Autodesk Inventor part; units mm, degrees
ref_plane "YZ Plane" through (0, 0, 0) normal (1, 0, 0) x (0, 1, 0)
ref_plane "XZ Plane" through (0, 0, 0) normal (0, 1, 0) x (-1, 0, 0)
ref_plane "XY Plane" through (0, 0, 0) normal (0, 0, 1) x (1, 0, 0)
sketch "Sketch1" plane through (0, 0, 0) normal (0, 1, 0) x (-1, 0, 0)
  line L0 (9.98, 16.98) -> (-9.98, 16.98)
  line L1 (-9.98, 16.98) -> (-9.98, -16.98)
  line L2 (-9.98, -16.98) -> (9.98, -16.98)
  line L3 (9.98, -16.98) -> (9.98, 16.98)
  line L4 (9.98, 16.98) -> (-9.98, -16.98) construction
  line L5 (-9.98, 16.98) -> (9.98, -16.98) construction
  point P0 (0, 0)
  dimension "d0" = 33.96
  dimension "d1" = 19.96
extrude "arm-horn" add sketch "Sketch1" along normal blind 3.3
fillet "Fillet1" radius 2 1 edges at (-9.98, 1.65, 16.98)
fillet "Fillet2" radius 2 1 edges at (9.98, 1.65, 16.98)
fillet "Fillet3" radius 2 1 edges at (9.98, 1.65, -16.98)
fillet "Fillet4" radius 2 1 edges at (-9.98, 1.65, -16.98)
sketch "Sketch3" plane through (0, 0, 0) normal (0, -1, 0) x (1, 0, 0)
  arc A0 (-2.612, 2.76) -> (-2.8345, 2.5309) centre (0, 0) ccw construction
  arc A1 (-1.9951, -14.4406) -> (1.9951, -14.4406) centre (0, -14.3) ccw
  arc A2 (0, 12.3) -> (1.9951, 14.4406) centre (0, 14.3) ccw construction
  line L0 (1.9951, 14.4406) -> (2.8345, 2.5309)
  line L1 (-1.9951, 14.4406) -> (-2.8345, 2.5309)
  line L2 (-2.8345, -2.5309) -> (-1.9951, -14.4406)
  line L3 (2.8345, -2.5309) -> (1.9951, -14.4406)
  circle A3 centre (0, -1.5) radius 2.9 construction
  arc A4 (-2.612, 2.76) -> (-2.8928, 1.7039) centre (0, 1.5) ccw construction
  line L4 (-7.98, 16.98) -> (7.98, 16.98) construction
  line L5 (0, 16.98) -> (0, -18.0608) construction
  line L6 (7.98, -16.98) -> (-7.98, -16.98) construction
  arc A5 (0, 4.4) -> (-2.612, 2.76) centre (0, 1.5) ccw construction
  arc A6 (2.612, 2.76) -> (0, 4.4) centre (0, 1.5) ccw construction
  arc A7 (0, 3.8) -> (-2.612, 2.76) centre (0, 0) ccw construction
  arc A8 (2.612, 2.76) -> (0, 3.8) centre (0, 0) ccw construction
  arc A9 (-2.8928, 1.7039) -> (-2.4819, 0) centre (0, 1.5) ccw construction
  arc A10 (-2.4819, 0) -> (2.4819, 0) centre (0, 1.5) ccw construction
  arc A11 (2.4819, 0) -> (2.8928, 1.7039) centre (0, 1.5) ccw construction
  arc A12 (2.8928, 1.7039) -> (2.612, 2.76) centre (0, 1.5) ccw construction
  line L7 (-2.8345, 2.5309) -> (-2.8928, 1.7039) construction
  arc A13 (-2.8345, 2.5309) -> (-2.8345, -2.5309) centre (0, 0) ccw
  arc A14 (0, -3.8) -> (2.612, -2.76) centre (0, 0) ccw construction
  arc A15 (-2.612, -2.76) -> (0, -3.8) centre (0, 0) ccw construction
  arc A16 (2.612, -2.76) -> (2.8345, -2.5309) centre (0, 0) ccw construction
  arc A17 (-2.8345, -2.5309) -> (-2.612, -2.76) centre (0, 0) ccw construction
  arc A18 (2.8345, -2.5309) -> (2.612, 2.76) centre (0, 0) ccw
  arc A19 (-1.9951, 14.4406) -> (0, 12.3) centre (0, 14.3) ccw construction
  arc A20 (1.9951, 14.4406) -> (-1.9951, 14.4406) centre (0, 14.3) ccw
  arc A21 (0, -12.3) -> (-1.9951, -14.4406) centre (0, -14.3) ccw construction
  arc A22 (1.9951, -14.4406) -> (0, -12.3) centre (0, -14.3) ccw construction
  line L8 (2.8345, 2.5309) -> (2.8928, 1.7039) construction
  point P0 (0, -16.98)
  dimension "d12" = 4
  dimension "d13" = 5.8
  dimension "d14" = 7.6
  dimension "d16" = 1.5
  dimension "d17" = 1.5
  dimension "d18" = 14.3
  dimension "d19" = 14.3
extrude "Extrusion3" cut sketch "Sketch3" against normal blind 2
sketch "Sketch6" plane through (0, 3.3, 0) normal (0, 1, 0) x (1, 0, 0)
  circle A0 centre (0, 0) radius 1
  circle A1 centre (0, 0) radius 1.5
  dimension "d29" = 2
  dimension "d30" = 3
extrude "Extrusion6" add sketch "Sketch6" against normal blind 2.2
sketch "Sketch7" plane through (0, 3.3, 0) normal (0, 1, 0) x (1, 0, 0)
  circle A0 centre (0, 0) radius 2.5
  dimension "d33" = 5
extrude "Extrusion7" cut sketch "Sketch7" against normal blind 1
sketch "Sketch8" plane through (0, 2.3, 0) normal (0, 1, 0) x (1, 0, 0)
  circle A0 centre (0, 0) radius 1
  dimension "d36" = 2
extrude "Extrusion8" cut sketch "Sketch8" against normal up to next
equation "\"d8\" = cornerrad"
equation "\"d9\" = cornerrad"
equation "\"d10\" = cornerrad"
equation "\"d11\" = cornerrad"
equation "\"d20\" = armslotd"
equation "\"printer3dtolerance\" = 0.1"
equation "\"wallw\" = 42"
equation "\"wallh\" = 44"
equation "\"cornerrad\" = 2"
equation "\"baseextra\" = 2"
equation "\"wall1_thick\" = 8"
equation "\"wall2_thick\" = 6.4"
equation "\"wall3_thick\" = 4"
equation "\"wall1slot\" = 8.1"
equation "\"wall2slot\" = 6.5"
equation "\"wall3slot\" = 4.1"
equation "\"gap2\" = 28"
equation "\"baseh\" = 79"
equation "\"basew\" = 44"
equation "\"base_thick\" = 6"
equation "\"base_slots_depth\" = 4"
equation "\"servobigcircledia\" = 11.6"
equation "\"servosmallcircledia\" = 5.9"
equation "\"servo9gw\" = 22.8"
equation "\"servomounth\" = 4"
equation "\"servomountsquare\" = 4"
equation "\"servopolygonr\" = 6.1"
equation "\"servopolygonl\" = 5.9"
equation "\"distancefrombottom\" = 34"
equation "\"distancefromleft\" = 22"
equation "\"wall3slotd\" = 2"
equation "\"wall3slotw\" = 36"
equation "\"adapterh\" = 16"
equation "\"adapterw\" = 32"
equation "\"armw\" = 34"
equation "\"armslotd\" = 2"
equation "\"armthick\" = 3"
equation "\"fanhs\" = 9.6"
equation "\"fanhb\" = 11"
equation "\"adapterwallthick\" = 6"
equation "\"adapterwallslotd\" = 2"
equation "\"armhornthick\" = 3"
equation "\"hornscrewholed\" = 2"
equation "\"hornthick\" = 1.5"
equation "\"hornscrewheadd\" = 3"
properties part number "arm-slot"
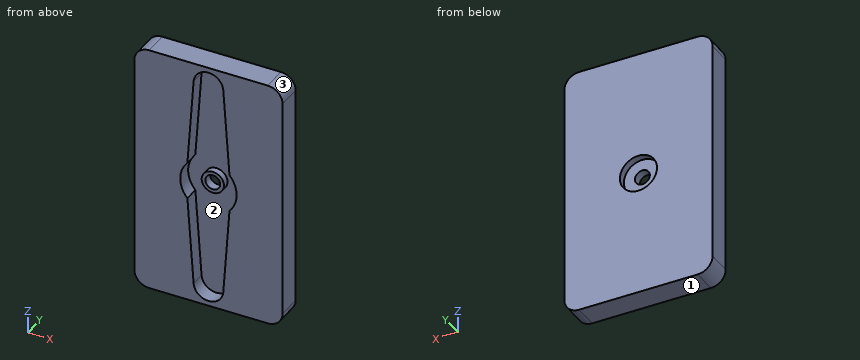
Read the model definition and answer for the solid it produces. Units are mm, in the model's axes. Face numbers are marked on the shaded views. Give positions to 0.01 mm unless a question says otherwise; leave off trailing zeros. Write each loop counter-clockwise with the first axis right and the second up, starting at its lowest first coordinate (ties: lowest second). Pieces come first, ordered by that corner, then holes. Notation, with made-up numbers: M -2,41.25 L 9,41.25 A29 ccw 9,68.25 Z; hole C 79,72 d11. An arc over 180 degrees is marked long. One line per item, written item: value. Start each with the question number.
(1) Find the intervals of material crossed by line 1 (X direction, y = 1.6, z = 0); line 2 (Z direction, x = 0, y = 1.7); line 3 (X direction, y = 1.4, z = 14.5), in increasing order.
(2) Find section D-D (x = -3.25). Determine the outline of the cut face in (y, z).
(3) Determine the mould class of the marked faces 1, 2 and 3 for opening direction X: pulls with the +X half, pulls with the -X half, needs draft (parallel to the pull), parting line crosses it, or undercut.
(4) Find section B-B (y = 1.55). Determine the outline of the cut face in (x, z), plus the area to 3 significant figures.
(5) Flat-ended cylindrical pins translate along their axes: pin 1 Ø3 at (x, z) = (0, 0) entering from +Y; pin 2 Ø0.9 at (x, z) = (0.5, -0.5) entering from -Y; pin 3 Ø1.2 at (x, z) = (0, 0) entering from -Y. Find the tip coordinate at first contact, or state that the pin passes through.
(6) Find section A-A (x = 0). Determine the outline of the cut face in (y, z), plus the area to 3 significant figures.
(7) Find section C-C (z = 0). Determine the outline of the cut face in (x, y).
Results below:
1. line 1: x = -9.98 to -3.8, -1.5 to -1, 1 to 1.5, 3.8 to 9.98
1. line 2: z = -16.98 to -16.3, -1.5 to -1, 1 to 1.5, 16.3 to 16.98
1. line 3: x = -9.98 to -1.99, 1.99 to 9.98
2. outline: M 0,-16.98 L 3.3,-16.98 L 3.3,16.98 L 0,16.98 L 0,1.97 L 2,1.97 L 2,-1.97 L 0,-1.97 Z
3. face 1: needs draft
3. face 2: undercut
3. face 3: pulls with the +X half
4. outline: M -9.98,-14.98 A2 ccw -7.98,-16.98 L 7.98,-16.98 A2 ccw 9.98,-14.98 L 9.98,14.98 A2 ccw 7.98,16.98 L -7.98,16.98 A2 ccw -9.98,14.98 Z; C 0,0 d3; hole M -2.83,-2.53 L -2,-14.44 A2 ccw 2,-14.44 L 2.83,-2.53 A3.8 ccw 2.83,2.53 L 2,14.44 A2 ccw -2,14.44 L -2.83,2.53 A3.8 ccw Z; hole C 0,0 d2
4. area: 516 mm^2
5. pin 1: stops at y = 2.3
5. pin 2: stops at y = 1.1
5. pin 3: passes through
6. outline: M 0,-16.98 L 3.3,-16.98 L 3.3,-2.5 L 2.3,-2.5 L 2.3,-1 L 1.1,-1 L 1.1,-1.5 L 2,-1.5 L 2,-16.3 L 0,-16.3 Z; M 0,16.3 L 2,16.3 L 2,1.5 L 1.1,1.5 L 1.1,1 L 2.3,1 L 2.3,2.5 L 3.3,2.5 L 3.3,16.98 L 0,16.98 Z
6. area: 42.2 mm^2
7. outline: M -9.98,0 L -3.8,0 L -3.8,2 L -1.5,2 L -1.5,1.1 L -1,1.1 L -1,2.3 L -2.5,2.3 L -2.5,3.3 L -9.98,3.3 Z; M 1,1.1 L 1.5,1.1 L 1.5,2 L 3.8,2 L 3.8,0 L 9.98,0 L 9.98,3.3 L 2.5,3.3 L 2.5,2.3 L 1,2.3 Z
